Geometry: final body of the model. Coordinates: model frame, mm. A direction names the side the tool comes from. Coordinates: 2 decimals unless noted, no trailing zeros. Order: outer loops, then holes, each group sorted by start corner. A loop starts at its lowest first (then second) coordinate and runs counter-clockwise, first axis right, second up. Notation, with made-up numbers: (55, -4) - (101, -4) arc R11 cw to (101, 1) - close; hole circle Ø2 at (84.25, -35). An arc over 180 degrees is marked (long way). Use a Markdown table: item, result. Add a question column.
```python
from build123d import *

# Parameters (mm, degrees)
F0_R     = 50
F1_DEPTH = 80
F2_R     = 15
F3_DEPTH = 80.001
F4_R     = 9
F5_DEPTH = 25
F7_D     = 10
F7_DEPTH = 20
F7_TIP   = 3.0043030951


with BuildPart() as f1:
    # F0 (on Top) → F1 (new body)
    with BuildSketch(Plane.XY):
        Circle(F0_R)
    extrude(amount=F1_DEPTH)

    # F2 (on face) → F3 (cut, through all)
    with BuildSketch(Plane.XY.offset(80)):
        with Locations((0, 30)):
            Circle(F2_R)
        with Locations((-30, 0)):
            Circle(F2_R)
        with Locations((0, -30)):
            Circle(F2_R)
        with Locations((30, 0)):
            Circle(F2_R)
    extrude(amount=-F3_DEPTH, mode=Mode.SUBTRACT)

    # F4 (on face) → F5 (join)
    with BuildSketch(Plane(origin=(0, 0, 0), x_dir=(1, 0, 0), z_dir=(0, 0, -1))):
        Circle(F4_R)
    extrude(amount=F5_DEPTH)

    # F7
    with Locations(Plane(origin=(0, 0, -25), x_dir=(1, 0, 0), z_dir=(0, 0, -1))):
        with Locations((0, 0)):
            Hole(F7_D / 2, depth=F7_DEPTH)
            with Locations((0, 0, -(F7_DEPTH + F7_TIP / 2))):  # 118° drill point
                Cone(0, F7_D / 2, F7_TIP, mode=Mode.SUBTRACT)


solid = f1.part
```
1) Line query: line 1 (Y direction, x = 0, z = 20.5); line 2 (Y direction, x = 1.5, z = 17.5); line 3 (Y direction, x = 0, z = -18). Output: solid intervals per line, ascending. Write a range as from..to.
2) Section query A-A (x = -30). Return the cut outline in (y, z), and give its area (3 significant figures).
3) Section query C-C (z = -8.5). Return the cut outline in (x, y), and give its area (3 significant figures).
4) Section query B-B (y = -32). Return the cut outline in (x, z).
5) Draft query along X for faces 1 (the cylindrical face through (47.69, 15.02, 39.44)), 2 (the flat face through (-1, 1, 80)), 3 (the cylindrical face through (15.015, 0.66, 40.56)). Return one class per face: released by +X, released by -X, zero draft, split by the parting line, or undercut.
6) Access query for faces 4 (the cylindrical face through (-1.172, -8.923, -12.325)), 5 (the cylindrical face through (-44.985, 0.66, 40.56)). Directions: +Z, -Z, +X, -X, +Y, -Y. A direction counts if a zero-diameter tool reaches every point of the face in a straight line with its end or side. Return the directions, or none.
7) First-contact query: pin 1 (6 mm diameter, centred on x = -28, z = -5.5, fed in from -Y); pin 2 (1.5 mm diameter, centred on x = -34.5, z = 26, fed in from -Y); pin 3 (12 mm diameter, centred on x = 11.5, z = 44.5, fed in from -Y); pin 4 (4 mm diameter, centred on x = -14, z = 22, fed in from -Y). Flat tips, straight axial feed; report the tip coordinate or a pass-through.
8) Section query D-D (z = 33). Return the cut outline in (x, y).
From the geometry:
| question | item | result |
|---|---|---|
| 1 | line 1 | y = -50..-45, -15..15, 45..50 |
| 1 | line 2 | y = -49.98..-44.92, -15.08..15.08, 44.92..49.98 |
| 1 | line 3 | y = -9..-5, 5..9 |
| 2 | outline | (-40, 0) - (-15, 0) - (-15, 80) - (-40, 80) - close; (15, 0) - (40, 0) - (40, 80) - (15, 80) - close |
| 2 | area | 4,000 mm^2 |
| 3 | outline | circle Ø18 at (0, 0); hole circle Ø10 at (0, 0) |
| 3 | area | 176 mm^2 |
| 4 | outline | (-38.42, 0) - (-14.87, 0) - (-14.87, 80) - (-38.42, 80) - close; (14.87, 0) - (38.42, 0) - (38.42, 80) - (14.87, 80) - close |
| 5 | face 1 | split by the parting line |
| 5 | face 2 | zero draft |
| 5 | face 3 | undercut |
| 6 | face 4 | -Z |
| 6 | face 5 | +Z, -Z |
| 7 | pin 1 | passes through |
| 7 | pin 2 | stops at y = -36.89 |
| 7 | pin 3 | stops at y = -49.7 |
| 7 | pin 4 | stops at y = -48.54 |
| 8 | outline | circle Ø100 at (0, 0); hole circle Ø30 at (-30, 0); hole circle Ø30 at (0, -30); hole circle Ø30 at (0, 30); hole circle Ø30 at (30, 0) |
